from build123d import *

# Parameters (mm, degrees)
F1_DEPTH = 44.45
F2_SIZE  = 12.7
F3_W     = 15.875
F3_H     = 6.35
F4_DEPTH = 241.3


with BuildPart() as f1:
    # F0 (on Front) → F1 (new body, symmetric)
    with BuildSketch(Plane.XZ):
        Polygon((228.6, -20.6375), (228.6, 20.6375), (139.7, 20.6375), (139.7, 52.3875), (-146.05, 52.3875), (-146.05, 20.6375), (-228.6, 20.6375), (-228.6, -20.6375), align=None)
    extrude(amount=F1_DEPTH, both=True)

    # F2
    f2_edges = [f1.edges().sort_by_distance(p)[0] for p in [
        (-146.05, 0, 52.3875),
        (-228.6, 0, 20.6375),
        (139.7, 0, 52.3875),
        (228.6, 0, 20.6375),
    ]]
    chamfer(f2_edges, length=F2_SIZE)

    # F3 (on Right) → F4 (cut, symmetric)
    with BuildSketch(Plane.YZ):
        with Locations((-23.8125, -17.4625)):
            Rectangle(F3_W, F3_H)
        with Locations((23.8125, -17.4625)):
            Rectangle(F3_W, F3_H)
    extrude(amount=F4_DEPTH, both=True, mode=Mode.SUBTRACT)


solid = f1.part
Geometry: final body of the model. Coordinates: model frame, mm. A direction names the side the tool comes from. Round coordinates to 2 decimals unless told otherwise and drop trailing zeros. Loops run counter-clockwise (first coordinate to the right, second up) from the corner with the lowest first, then second, coordinate; pieces in that order, holes last. Notation, with made-up numbers: M 74,-6 L 92,-6 A36 ccw 92,29 Z; hole C -28.75,-9 d1. An arc over 180 degrees is marked long. One line per question, with ' | ' between items.
(1) Material intervals for line 1 along Y through (x, z) = (75, -14.5) (3 decimals); line 2 along Z through (x, y) = (124.5, -31.5); line 3 along X through (y, z) = (31.5, 45.5), sorted ascending. Write a range as from..to.
Check result:
line 1: y = -44.45..-31.75, -15.875..15.875, 31.75..44.45 | line 2: z = -14.29..52.39 | line 3: x = -140.24..133.89
(2) Pull-direction query (Z, two-part tool) for faces 1 (the flat face through (-180, -1, 20.638)), 2 (the flat face through (-228.6, -1, -6)), 3 (the flat face through (-3, 38, -20.638)); classes: +Z half, -Z half, draft (parallel to the pull), parting line (faces both ways), or undercut.
Check result:
face 1: +Z half | face 2: draft | face 3: -Z half
(3) Contact query for flat-ended pins moving along their axis: P1, Ø5, axis at y = 19, z = 41.5, coming from the +X side; P2, Ø9.5, axis at y = -0.5, z = 29, coming from the -X side; P3, Ø1.5, axis at x = 172.5, y = -22, coming from the -Z side. Output: stop coordinate, or through.
Check result:
P1: stops at x = 139.7 | P2: stops at x = -146.05 | P3: stops at z = -14.29
(4) Access query for faces 4 (the flat face through (178, -1, 20.638)), 5 (the flat face through (-146.05, -1, 30)), 6 (the flat face through (3, 24, -14.287)), 7 (the flat face through (-3, 0, -20.638)). Directions: +Z, -Z, +X, -X, +Y, -Y. A direction counts if a zero-diameter tool reaches every point of the face in a straight line with its end or side. Return the directions, or none.
Check result:
face 4: +Z, +X, +Y, -Y | face 5: +Z, -X, +Y, -Y | face 6: -Z, +X, -X | face 7: -Z, +X, -X, +Y, -Y
(5) Cut plane C-C on z = 28. Return the cut outline in (x, y), plus the area to 3 significant figures.
Check result:
outline: M -146.05,-44.45 L 139.7,-44.45 L 139.7,44.45 L -146.05,44.45 Z | area: 25,400 mm2
(6) Cut plane B-B on y = 27. Return the cut outline in (x, z).
Check result:
outline: M -228.6,-14.29 L 228.6,-14.29 L 228.6,7.94 L 215.9,20.64 L 139.7,20.64 L 139.7,39.69 L 127,52.39 L -133.35,52.39 L -146.05,39.69 L -146.05,20.64 L -215.9,20.64 L -228.6,7.94 Z
